```python
from build123d import *

# Parameters (mm, degrees)
F1_DEPTH = 7


with BuildPart() as f1:
    # F0 (on Top) → F1 (new body)
    with BuildSketch(Plane.XY):
        with BuildLine():
            Line((-25.475699, 40.335676), (-25.475699, 45.835676))
            Line((-25.475699, 45.835676), (-21.075699, 45.835676))
            Line((-21.075699, 45.835676), (-21.075699, 33.835676))
            Line((-21.075699, 33.835676), (-21.075699, 31.835676))
            Line((-21.075699, 31.835676), (-19.6757, 31.835676))
            Line((-19.6757, 31.835676), (-19.6757, 33.835676))
            Line((-19.6757, 33.835676), (-19.6757, 37.435679))
            Line((-19.6757, 37.435679), (-17.6757, 39.435679))
            ThreePointArc((-17.6757, 39.435679), (-14.89494, 38.638502), (-13.013308, 40.835677))
            Line((-13.013308, 40.835677), (-14.946623, 40.835677))
            ThreePointArc((-14.946623, 40.835677), (-15.664693, 40.460677), (-16.382763, 40.835677))
            Line((-16.382763, 40.835677), (-19.6757, 40.835677))
            Line((-19.6757, 40.835677), (-19.6757, 41.835677))
            Line((-19.6757, 41.835677), (-16.382763, 41.835677))
            ThreePointArc((-16.382763, 41.835677), (-15.664693, 42.210677), (-14.946623, 41.835677))
            Line((-14.946623, 41.835677), (-13.013308, 41.835677))
            ThreePointArc((-13.013308, 41.835677), (-13.230669, 42.582711), (-13.653686, 43.235675))
            ThreePointArc((-13.653686, 43.235675), (-15.664693, 44.145927), (-17.6757, 43.235675))
            Line((-17.6757, 43.235675), (-19.6757, 45.235675))
            Line((-19.6757, 45.235675), (-19.6757, 47.235675))
            Line((-19.6757, 47.235675), (-26.875699, 47.235675))
            Line((-26.875699, 47.235675), (-26.875699, 38.935676))
            Line((-26.875699, 38.935676), (-25.758563, 38.935676))
            Line((-25.758563, 38.935676), (-25.299585, 33.689533))
            Line((-25.299585, 33.689533), (-25.125273, 31.697143))
            Line((-25.125273, 31.697143), (-23.730601, 31.819161))
            Line((-23.730601, 31.819161), (-23.904913, 33.811551))
            Line((-23.904913, 33.811551), (-24.475699, 40.335676))
            Line((-24.475699, 40.335676), (-25.475699, 40.335676))
        make_face()
    extrude(amount=F1_DEPTH)


solid = f1.part
```
Build history of the part. All positions in model axes, mm. A direction names the side the tool comes from. Round coordinates to 2 decimals unless told otherwise and drop trailing zeros. Loops run counter-clockwise (first coordinate to the right, second up) from the corner with the lowest first, then second, coordinate; pieces in that order, holes last.
Item 1: Drill centre lines: line 1 along X through (y, z) = (43.5, 4); line 2 along Y through (x, z) = (-15.75, 3.75); line 3 along X through (y, z) = (38.75, 3.5). Where is each one in solid material? Low to high.
Item 2: Two-plate mould, pull along X, no slides. Class faces 6 (the face through (-18.69, 38.42, 3.45)), 7 (the face through (-19.676, 41, 3)), 8 (the face through (-14, 41.836, 3)): released by +X, released by -X, zero draft, split by the parting line, or undercut.
Item 3: Saw through at D-D (z = 0.75). List the corners of the cut face in (x, y) (3 decimals), then the cut area to 3 significant figures.
Item 4: Saw through at A-A (y = 41.5). List the corners of the cut face in (x, z), then the cut area to 3 significant figures.
Item 5: Saw through at C-C (y = 43.75). List the corners of the cut face in (x, z).
Item 6: Pin check, flat tips, straight feed: P1, Ø2, axis at x = -24.5, z = 3.5, coming from the -Y side; P2, Ø3, axis at y = 36, z = 2.5, coming from the -X side; P3, Ø3.5, axis at x = -22.5, z = 2, coming from the -Y side; P4, Ø2, axis at y = 46, z = 2.5, coming from the +X side. Stop position of each tip, or through.
Item 7: Which spindle directions (+Z, -Z, +X, -X, +Y, -Y) get a long thin tool onto all of the face, cutting with end or side? Do faces 1 (the face through (-18.66, 44.22, 3.45)), 2 (the face through (-19.676, 46, 3)), 3 (the face through (-18, 40.836, 3)), 4 (the face through (-15.68, 42.21, 3.45)), 5 (the face through (-26, 38.936, 3)). Say none if no direction does.
Item 8: Saw through at B-B (x = -17). List the corners of the cut face in (y, z).
Worked answers:
1. line 1: x = -26.88 to -25.48, -21.08 to -17.94, -17.41 to -13.92
1. line 2: y = 38.53 to 40.46, 42.21 to 44.14
1. line 3: x = -25.74 to -24.34, -21.08 to -18.36, -16.74 to -14.59
2. face 6: undercut
2. face 7: released by +X
2. face 8: zero draft
3. outline: (-26.876, 38.936) - (-25.759, 38.936) - (-25.3, 33.69) - (-25.125, 31.697) - (-23.731, 31.819) - (-23.905, 33.812) - (-24.476, 40.336) - (-25.476, 40.336) - (-25.476, 45.836) - (-21.076, 45.836) - (-21.076, 31.836) - (-19.676, 31.836) - (-19.676, 37.436) - (-17.676, 39.436) arc R2.677 ccw to (-13.013, 40.836) - (-14.947, 40.836) arc R0.875 cw to (-16.383, 40.836) - (-19.676, 40.836) - (-19.676, 41.836) - (-16.383, 41.836) arc R0.875 cw to (-14.947, 41.836) - (-13.013, 41.836) arc R2.677 ccw to (-13.654, 43.236) arc R2.677 ccw to (-17.676, 43.236) - (-19.676, 45.236) - (-19.676, 47.236) - (-26.876, 47.236) - close
3. area: 77.2 mm2
4. outline: (-26.88, 0) - (-25.48, 0) - (-25.48, 7) - (-26.88, 7) - close; (-21.08, 0) - (-19.68, 0) - (-19.68, 7) - (-21.08, 7) - close
4. area: 19.6 mm2
5. outline: (-26.88, 0) - (-25.48, 0) - (-25.48, 7) - (-26.88, 7) - close; (-21.08, 0) - (-18.19, 0) - (-18.19, 7) - (-21.08, 7) - close; (-17.07, 0) - (-14.26, 0) - (-14.26, 7) - (-17.07, 7) - close
6. P1: stops at y = 31.7
6. P2: stops at x = -25.63
6. P3: stops at y = 31.77
6. P4: stops at x = -19.44
7. face 1: +Z, -Z, +Y
7. face 2: +Z, -Z, +X, +Y
7. face 3: +Z, -Z, +X
7. face 4: +Z, -Z
7. face 5: +Z, -Z, -X, -Y
8. outline: (38.88, 0) - (40.84, 0) - (40.84, 7) - (38.88, 7) - close; (41.84, 0) - (43.79, 0) - (43.79, 7) - (41.84, 7) - close
